Can you work these out from the model? Positions are in its coordinate system, mm. A direction names the side the tool comes from. Round coordinates to 2 decimals unless told otherwise and drop trailing zeros. Loops run counter-clockwise (first coordinate to the right, second up) from the corner with the lowest first, then second, coordinate; pieces in that order, holes last. Notation, with made-up numbers: M 76,53 L 109,53 A14 cw 109,61 Z; hole C -4,-30 d5. An arc over 180 degrees is marked long. Answer as CSV lines item,"result".
Autodesk Inventor part; units mm, degrees
ref_plane "YZ Plane" through (0, 0, 0) normal (1, 0, 0) x (0, 1, 0)
ref_plane "XZ Plane" through (0, 0, 0) normal (0, 1, 0) x (-1, 0, 0)
ref_plane "XY Plane" through (0, 0, 0) normal (0, 0, 1) x (1, 0, 0)
sketch "Sketch1" plane through (0, 0, 0) normal (0, 0, 1) x (1, 0, 0)
  line L0 (0, 0) -> (46.863, 0)
  line L1 (46.863, 0) -> (46.863, 38.1)
  line L2 (46.863, 38.1) -> (0, 38.1)
  line L3 (0, 38.1) -> (0, 0)
  dimension "d0" = 46.863
  dimension "d1" = 38.1
extrude "Extrusion1" add sketch "Sketch1" along normal blind 6.35
sketch "Sketch2" plane through (0, 0, 6.35) normal (0, 0, 1) x (1, 0, 0)
  line L0 (46.863, 38.1) -> (0, 38.1)
  line L1 (0, 0) -> (46.863, 0)
  line L2 (0, 38.1) -> (6.35, 38.1)
  line L3 (6.35, 38.1) -> (6.35, 0)
  line L4 (6.35, 0) -> (0, 0)
  line L5 (0, 0) -> (0, 38.1)
  dimension "d4" = 6.35
extrude "Extrusion2" add sketch "Sketch2" along normal blind 12.7
sketch "Sketch4" plane through (0, 0, 6.35) normal (0, 0, 1) x (1, 0, 0)
  line L0 (46.863, 38.1) -> (6.35, 38.1)
  line L1 (46.863, 0) -> (46.863, 38.1)
  point P0 (0, 0)
  point P1 (41.783, 30.2768)
  point P2 (40.513, 38.1)
  point P3 (6.35, 38.1)
  point P4 (43.688, 3.175)
  point P5 (43.688, 34.925)
  dimension "d8" = 7.8232
  dimension "d9" = 5.08
hole "Hole1" at (41.783, 30.2768, 6.35) direction (0, 0, -1) diameter 4.572 end through all
sketch "Sketch5" plane through (0, 0, 6.35) normal (0, 0, 1) x (1, 0, 0)
  line L0 (6.35, 0) -> (46.863, 0)
  line L1 (46.863, 0) -> (46.863, 38.1)
  point P0 (0, 0)
  point P1 (41.783, 7.8232)
  point P2 (6.35, 0)
  point P3 (40.513, 0)
  point P4 (43.688, 3.175)
  point P5 (43.688, 34.925)
  dimension "d17" = 7.8232
  dimension "d18" = 5.08
hole "Hole2" at (41.783, 7.8232, 6.35) direction (0, 0, -1) diameter 4.572 end through all
sketch "Sketch6" plane through (6.35, 0, 6.35) normal (1, 0, 0) x (0, 0, -1)
  line L0 (-12.7, 0) -> (-12.7, 38.1)
  line L1 (0, 38.1) -> (-12.7, 38.1)
  point P0 (6.35, 0)
  point P1 (-6.35, 31.75)
  dimension "d26" = 6.35
  dimension "d27" = 6.35
hole "Hole3" at (6.35, 31.75, 12.7) direction (-1, 0, 0) diameter 5.0038 end through all
sketch "Sketch7" plane through (6.35, 0, 6.35) normal (1, 0, 0) x (0, 0, -1)
  line L0 (-12.7, 0) -> (-12.7, 38.1)
  line L1 (0, 0) -> (-12.7, 0)
  point P0 (6.35, 0)
  point P1 (-6.35, 6.35)
  dimension "d35" = 6.35
  dimension "d36" = 6.35
hole "Hole4" at (6.35, 6.35, 12.7) direction (-1, 0, 0) diameter 5.0038 end through all
fillet "Fillet3" radius 3.175 4 edges at (3.175, 38.1, 19.05) (3.175, 0, 19.05) (46.863, 38.1, 3.175) (46.863, 0, 3.175)
fillet "Fillet4" radius 1.5875 1 edges at (6.35, 19.05, 6.35)
sketch "Sketch8" plane through (0, 0, 6.35) normal (0, 0, 1) x (1, 0, 0)
  line L0 (46.863, 3.175) -> (46.863, 34.925)
  line L1 (43.688, 38.1) -> (7.9375, 38.1)
  point P0 (0, 0)
  point P1 (11.4046, 30.2768)
  dimension "d47" = 35.4584
  dimension "d48" = 7.8232
hole "Hole5" at (11.4046, 30.2768, 6.35) direction (0, 0, -1) diameter 4.572 end through all
sketch "Sketch9" plane through (0, 0, 6.35) normal (0, 0, 1) x (1, 0, 0)
  line L0 (7.9375, 0) -> (43.688, 0)
  line L1 (46.863, 3.175) -> (46.863, 34.925)
  point P0 (0, 0)
  point P1 (11.4046, 7.8232)
  dimension "d56" = 7.8232
  dimension "d57" = 35.4584
hole "Hole6" at (11.4046, 7.8232, 6.35) direction (0, 0, -1) diameter 4.572 end through all
sketch "Sketch10" plane through (0, 0, 6.35) normal (0, 0, 1) x (1, 0, 0)
  line L0 (22.3774, 17.78) -> (30.8356, 17.78) construction
  line L1 (26.6065, 17.78) -> (26.6065, 25.1206) construction
  line L2 (46.863, 3.175) -> (46.863, 34.925)
  line L3 (7.9375, 0) -> (43.688, 0)
  line L4 (22.3774, 11.43) -> (30.8356, 11.43)
  line L5 (32.1087, 28.2905) -> (36.3378, 20.9499)
  arc A0 (32.8202, 23.8119) -> (26.6065, 13.0432) centre (30.8356, 17.78) ccw construction
  arc A1 (30.8356, 11.43) -> (36.3378, 20.9499) centre (30.8356, 17.78) ccw
  line L6 (21.1043, 28.2905) -> (16.8752, 20.9499)
  arc A2 (26.6065, 13.0432) -> (20.3928, 23.8119) centre (22.3774, 17.78) ccw construction
  arc A3 (16.8752, 20.9499) -> (22.3774, 11.43) centre (22.3774, 17.78) ccw
  arc A4 (32.1087, 28.2905) -> (21.1043, 28.2905) centre (26.6065, 25.1206) ccw
  arc A5 (20.3928, 23.8119) -> (32.8202, 23.8119) centre (26.6065, 25.1206) ccw construction
  line L7 (20.0039, 28.9245) -> (15.7157, 21.618)
  arc A6 (15.7157, 21.618) -> (20.574, 10.3063) centre (22.3774, 17.78) ccw
  arc A7 (32.639, 10.3765) -> (37.4382, 21.5839) centre (30.8356, 17.78) ccw
  line L8 (37.4382, 21.5839) -> (33.2091, 28.9245)
  arc A8 (33.2091, 28.9245) -> (20.0039, 28.9245) centre (26.6065, 25.1206) ccw
  line L9 (20.574, 6.35) -> (32.639, 6.35)
  line L10 (26.6065, 6.35) -> (26.6065, 4.7621) construction
  line L11 (20.574, 6.35) -> (20.574, 10.3063)
  line L12 (32.639, 6.35) -> (32.639, 10.3765)
  point P0 (0, 0)
  dimension "d65" = 8.4582
  dimension "d71" = 7.3406
  dimension "d72" = 20.2565
  dimension "d73" = 17.78
  dimension "d74" = 1.27
  dimension "d75" = 11.43
  dimension "d76" = 12.065
  dimension "d77" = 0
extrude "Extrusion3" cut sketch "Sketch10" against normal through all contours A3 L6 A4 L5 A1 L4 | A8 L8 A7 L12 L9 L11 A6 L7
fillet "Fillet5" radius 1.5875 2 edges at (20.574, 6.35, 3.175) (32.639, 6.35, 3.175)
fillet "Fillet6" radius 1.5875 2 edges at (20.574, 10.3063, 3.175) (32.639, 10.3765, 3.175)
properties part number "CAN Resistor Mount"
Item 1: If we section it at D-D on z = 2.75: State how many separate pieces and enclosed holes the cut face has, then the cut area to 3 significant figures.
Output:
separate pieces,"1"
enclosed holes,"5"
area,"1,260 mm2"
Item 2: If we section it at A-A on z = 12.7: Write out the boundary of the cut face in (x, y).
Output:
outline,"M 0,0 L 6.35,0 L 6.35,3.85 L 0,3.85 Z; M 0,8.85 L 6.35,8.85 L 6.35,29.25 L 0,29.25 Z; M 0,34.25 L 6.35,34.25 L 6.35,38.1 L 0,38.1 Z"
Item 3: If I drill on line 1 along Y through (x, z) = (4.25, 12.7); line 2 along Y through (x, z) = (42, 1); line 3 along Y through (x, z) = (26.5, 2), over which ranges is the centre line in solid material (lowest first)? Write a range as from..to.
Output:
line 1,"y = 0..3.85, 8.85..29.25, 34.25..38.1"
line 2,"y = 0..5.55, 10.1..28, 32.55..38.1"
line 3,"y = 0..6.35, 32.74..38.1"
Item 4: We'd pull the mould along Y, two halves only. Please class faces 3 (the face through (46, 37.1, 3.2)), 4 (the face through (36, 28, 6.35)), 5 (the face through (43.8, 29.2, 3.1)): released by +Y, released by -Y, zero draft, split by the parting line, or undercut.
Output:
face 3,"released by +Y"
face 4,"zero draft"
face 5,"undercut"
Item 5: Will these pins go through, and if not, where does the flat tip stop? pin 1 (4 mm diameter, centred on y = 19.5, z = 15.5, fed in from +X); pin 2 (2.5 mm diameter, centred on x = 11.4, y = 30.28, fed in from +Z); pin 3 (19 mm diameter, centred on x = 20, y = 21, fed in from +Z).
Output:
pin 1,"stops at x = 6.35"
pin 2,"passes through"
pin 3,"stops at z = 6.35"
Item 6: If we section it at B-B on x = 5.5: Write out the boundary of the cut face in (y, z) (3 decimals).
Output:
outline,"M 0,0 L 38.1,0 L 38.1,15.875 A3.175 ccw 34.925,19.05 L 3.175,19.05 A3.175 ccw 0,15.875 Z; hole C 6.35,12.7 d5.004; hole C 31.75,12.7 d5.004"
Item 7: On a 3-axis mill with a long thin cutter (end or side, diameter ignored), from which of +Z, -Z, +X, -X, +Y, -Y can I reach the whole of each face in a straight line? I mean faces 1 (the face through (3.13, 37.15, 18.14)), 2 (the face through (20.29, 10.05, 3.13)). Say none if no direction works.
Output:
face 1,"+Z, +X, -X, +Y"
face 2,"+Z, -Z"
Item 8: If we section it at C-C on x = 36: Write out the boundary of the cut face in (y, z), then the cut area to 3 significant figures.
Output:
outline,"M 0,0 L 12.18,0 L 12.18,6.35 L 0,6.35 Z; M 24.08,0 L 38.1,0 L 38.1,6.35 L 24.08,6.35 Z"
area,"166 mm2"
